Could you check a few things on this model? Use its own coordinates, in mm. A direction names the side the tool comes from. Give positions to 0.01 mm unless a question says otherwise; leave off trailing zeros. Order: outer loops, then holes, each group sorted by start corner. A loop starts at its lowest first (then second) coordinate and runs counter-clockwise, first axis right, second up.
(1) Imagine slicing it at B-B, the plane x = 38.5. Write out the boundary of the cut face in (y, z).
(2) Imagine slicing it at D-D, the plane x = 6.5. Write out the boundary of the cut face in (y, z), then the cut area to 3 significant figures.
(3) Imagine slicing it at C-C, the plane z = 7.5. Write out the boundary of the cut face in (x, y), then the cut area to 3 significant figures.
(4) On a 3-axis mill with a long thin cutter (end or side, diameter ignored), from which of +Z, -Z, +X, -X, +Y, -Y can I reach the whole of each face in a straight line? I mean faces 1 (the flat face through (36, 0, 21)), 2 (the flat face through (19, -3, 42)), 3 (the flat face through (18, 11, 45)), 4 (the flat face through (18, 10, 47)). Say none if no direction works.
(5) Will these pins go through, and if not, where does the flat tip stop? pin 1 (7.5 mm diameter, centred on x = 24, y = 1.5, fed in from +Z); pin 2 (5 mm diameter, centred on x = 23.5, z = 3.5, fed in from -Y); pin 3 (3 mm diameter, centred on x = 15, y = 3, fed in from +Z).
(6) If we mould it in two halves opening along X, with no side actions, what happens to faces 5 (the flat face through (-5, 5, 22)), 6 (the flat face through (18, 10, 21)), 7 (the flat face through (18, -1, 45))? For each: released by +X, released by -X, zero draft, split by the parting line, or undercut.
(7) Imagine slicing it at A-A, the plane y = 10.75. Write out the boundary of the cut face in (x, z), then the cut area to 3 significant figures.
(8) If I drill on probe 1 along Z at (x, y) = (13.5, -2.5); probe 2 along Z at (x, y) = (16, -1); probe 3 along X at (y, z) = (1, 36.5), over which ranges is the centre line in solid material (lowest first)?
from build123d import *

# Parameters (mm, degrees)
EXTRUDE_1_DEPTH = 42
SKETCH_2_W      = 8
SKETCH_2_H      = 42
SKETCH_2_W_2    = 7
EXTRUDE_2_DEPTH = 5
SKETCH_3_W      = 47
SKETCH_3_H      = 20
EXTRUDE_3_DEPTH = 5
EXTRUDE_4_DEPTH = 47


with BuildPart() as part:
    # 스케치1 → 보스-돌출1 (new body)
    with BuildSketch(Plane.XY):
        Polygon((-5, 0), (0, 0), (0, 10), (37, 10), (37, 0), (42, 0), (42, 15), (-5, 15), align=None)
    extrude(amount=EXTRUDE_1_DEPTH)

    # 스케치2 → 보스-돌출2 (add)
    with BuildSketch(Plane.XZ):
        with Locations((-1, 21)):
            Rectangle(SKETCH_2_W, SKETCH_2_H)
        with Locations((38.5, 21)):
            Rectangle(SKETCH_2_W_2, SKETCH_2_H)
    extrude(amount=EXTRUDE_2_DEPTH)

    # 스케치3 → 보스-돌출3 (add)
    with BuildSketch(Plane(origin=(0, 0, 0), x_dir=(-1, 0, 0), z_dir=(0, 0, -1))):
        with Locations((-18.5, 5)):
            Rectangle(SKETCH_3_W, SKETCH_3_H)
    extrude(amount=EXTRUDE_3_DEPTH)

    # 스케치4 → 보스-돌출4 (add)
    with BuildSketch(Plane.ZY.offset(5)):
        Polygon((42, 15), (48, 15), (48, 10), (45, 10), (45, 12), (42, 12), align=None)
        Polygon((42, -5), (48, -5), (48, 0), (45, 0), (45, -2), (42, -2), align=None)
    extrude(amount=-EXTRUDE_4_DEPTH)


solid = part.part
Answer block:
1. outline: (-5, -5) - (15, -5) - (15, 48) - (10, 48) - (10, 45) - (12, 45) - (12, 42) - (-2, 42) - (-2, 45) - (0, 45) - (0, 48) - (-5, 48) - close
2. outline: (-5, -5) - (15, -5) - (15, 48) - (10, 48) - (10, 45) - (12, 45) - (12, 42) - (10, 42) - (10, 0) - (-5, 0) - close; (-5, 42) - (-2, 42) - (-2, 45) - (0, 45) - (0, 48) - (-5, 48) - close
2. area: 358 mm2
3. outline: (-5, -5) - (3, -5) - (3, 0) - (0, 0) - (0, 10) - (37, 10) - (37, 0) - (35, 0) - (35, -5) - (42, -5) - (42, 15) - (-5, 15) - close
3. area: 410 mm2
4. face 1: +Z
4. face 2: -Y
4. face 3: +X, -X
4. face 4: +Z, +X, -X
5. pin 1: stops at z = 48
5. pin 2: stops at y = 10
5. pin 3: stops at z = 0
6. face 5: released by -X
6. face 6: undercut
6. face 7: zero draft
7. outline: (-5, -5) - (42, -5) - (42, 42) - (-5, 42) - close; (-5, 45) - (42, 45) - (42, 48) - (-5, 48) - close
7. area: 2,350 mm2
8. probe 1: z = -5 to 0, 42 to 48
8. probe 2: z = -5 to 0, 45 to 48
8. probe 3: x = -5 to 0, 37 to 42
